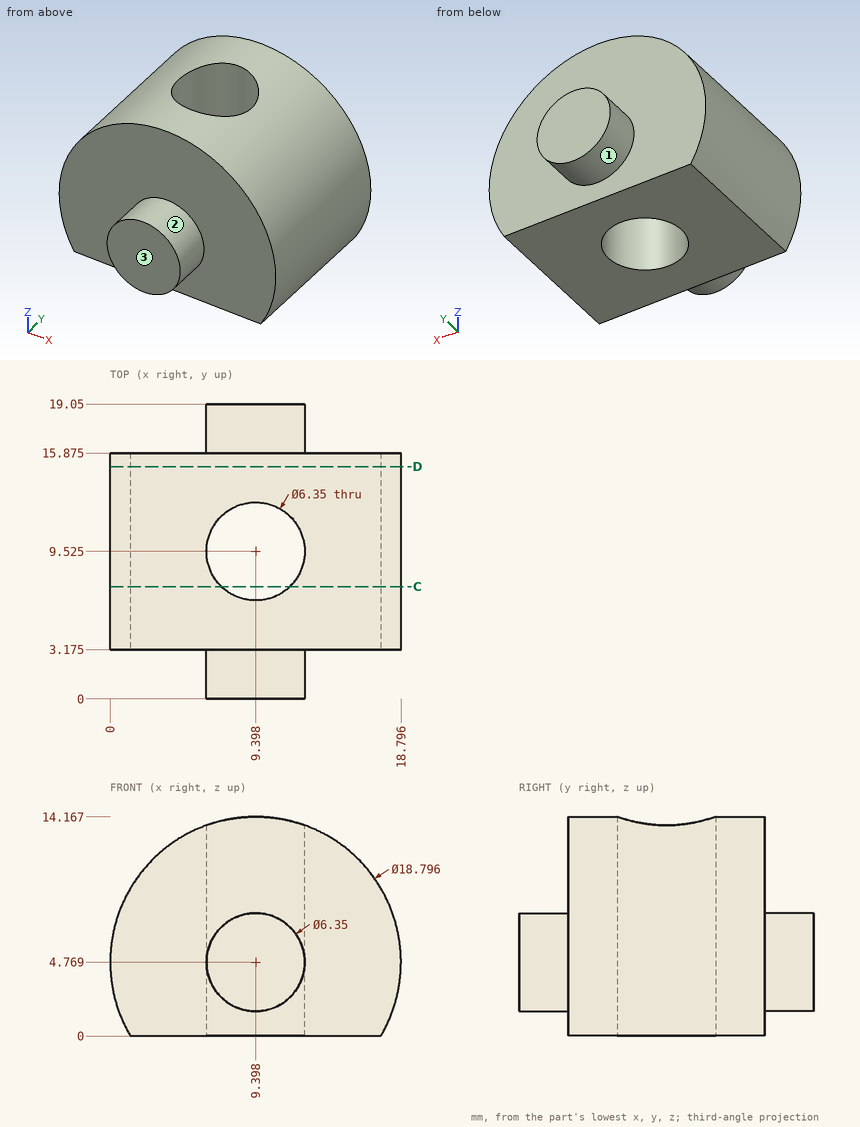
For this review, use the dimensioned drawing (mm, ordinates from the lowest corner) and the shaded views. A direction names the side the tool comes from. Coordinates: 2 decimals unless noted, no trailing zeros. Loops run counter-clockwise (first coordinate to the right, second up) from the corner with the lowest first, then second, coordinate; pieces in that order, holes last. Notation, with made-up numbers: (88, 37.5) -> (113, 37.5) arc R18 ccw to (113, 48.5) -> close; hole circle Ø4 at (-11, -2.5). An arc over 180 degrees is marked (long way). Use a Markdown table: item, result. Add a question column.
1. Machinability: for the marked faces 1, 2 and 3, which of the approach directions +Z, -Z, +X, -X, +Y, -Y give a long, thin tool a straight path to every point of the face, cutting with its end or side? Answer none if there is none.
2. Add section D-D on y = 15. Write out the cut boundary in (x, z).
3. Add section C-C on y = 7.25. Write out the cut boundary in (x, z), plus the area to 3 significant figures.
4. To check wall thickness, follow line 1 (X direction, y = 7.5, z = 2.25) (1 decimal); line 2 (Y direction, x = 16.25, z = 5.5) (1 decimal); line 3 (X direction, y = 8.75, z = 3.75) (1 decimal). State the ranges of each line that lie inside material, in increasing order.
5. Clearance check with a flat-ended pin moving along its axis: pin 1 Ø3 at (x, y) = (15.5, 3.5) entering from +Z. State where the tip first meets the part, or that it passes through.
Returned:
| question | item | result |
|---|---|---|
| 1 | face 1 | +Y |
| 1 | face 2 | -Y |
| 1 | face 3 | +Z, -Z, +X, -X, -Y |
| 2 | outline | (1.3, 0) -> (17.5, 0) arc R9.4 ccw (long way) to start |
| 3 | outline | (1.3, 0) -> (7.18, 0) -> (7.18, 13.9) arc R9.4 ccw to start; (11.61, 0) -> (17.5, 0) arc R9.4 ccw to (11.61, 13.9) -> close |
| 3 | area | 162 mm² |
| 4 | line 1 | x = 0.3 to 7, 11.8 to 18.5 |
| 4 | line 2 | y = 3.2 to 15.9 |
| 4 | line 3 | x = 0.1 to 6.3, 12.5 to 18.7 |
| 5 | pin 1 | stops at z = 12.96 |
